Verification items for the finished model (mm, model axes). A direction names the side the tool comes from. Give positions to 0.01 mm unless a question says otherwise; leave off trailing zeros. Loops run counter-clockwise (first coordinate to the right, second up) from the corner with the lowest first, then second, coordinate; pieces in that order, holes last. Notation, with made-up numbers: M 35,77 L 67,77 A22 ccw 67,86 Z; hole C -11,77 d6. An arc over 180 degrees is marked long. Use CSV: the item, a comma, the result in double quotes.
from build123d import *

# Parameters (mm, degrees)
F0_W     = 50.8
F0_H     = 50.8
F0_R     = 9.525
F1_DEPTH = 50.8
F2_DEPTH = 3.175
F3_R     = 2.38125
F4_DEPTH = 25.4
F5_W     = 4.124446
F5_H     = 1.190625
F6_DEPTH = 25.4
F7_R     = 3.175
F8_R     = 0.79375


with BuildPart() as f1:
    # F0 (on Front) → F1 (new body)
    with BuildSketch(Plane.XZ):
        Rectangle(F0_W, F0_H)
        Circle(F0_R, mode=Mode.SUBTRACT)
        Circle(F0_R)
    extrude(amount=-F1_DEPTH)

    # F0 (on Front) → F2 (join)
    with BuildSketch(Plane.XZ):
        Circle(F0_R)
    extrude(amount=F2_DEPTH)

    # F3 (on face) → F4 (join)
    with BuildSketch(Plane.XZ.offset(3.175)):
        Circle(F3_R)
    extrude(amount=F4_DEPTH)

    # F5 (on face) → F6 (cut, through all)
    with BuildSketch(Plane.XZ.offset(28.575)):
        with Locations((0, 1.785938)):
            Rectangle(F5_W, F5_H)
    extrude(amount=-F6_DEPTH, mode=Mode.SUBTRACT)

    # F7
    f7_edges = [f1.edges().sort_by_distance(p)[0] for p in [
        (25.4, 25.4, 25.4),
        (25.4, 25.4, -25.4),
        (-25.4, 25.4, 25.4),
        (-25.4, 25.4, -25.4),
    ]]
    fillet(f7_edges, radius=F7_R)

    # F8
    f8_edges = [f1.edges().sort_by_distance(p)[0] for p in [
        (0, 0, 25.4),
        (0, 50.8, 25.4),
        (-9.525, -3.175, 0),
    ]]
    fillet(f8_edges, radius=F8_R)


solid = f1.part
(1) Scan lines: L1, parallel to Y at x = 12.5, z = 18.5; L2, parallel to Y at x = 3.5, z = -4.5 (3 decimals); L3, parallel to Z at x = 23, y = 17.5. Record each from-to range of solid material in increasing order. Write a range as from..to.
Calculated:
L1,"y = 0..50.8"
L2,"y = -3.175..50.8"
L3,"z = -25.3..25.3"
(2) Section check B-B on z = 0. Record the cut outline in (x, y) (1 decimal).
Calculated:
outline,"M -25.4,0.8 A0.8 ccw -24.6,0 L -9.5,0 L -9.5,-2.4 A0.8 ccw -8.7,-3.2 L -2.4,-3.2 L -2.4,-28.6 L 2.4,-28.6 L 2.4,-3.2 L 8.7,-3.2 A0.8 ccw 9.5,-2.4 L 9.5,0 L 24.6,0 A0.8 ccw 25.4,0.8 L 25.4,50 A0.8 ccw 24.6,50.8 L -24.6,50.8 A0.8 ccw -25.4,50 Z"
(3) Tool access check on faces 1 (the flat face through (0, -16, 1.191)), 2 (the cylindrical face through (-7.559, -1.174, -5.796)), 3 (the flat face through (-25.4, 25, 0)). Record the directions out of +Z, -Z, +X, -X, +Y, -Y that give a thin tool (end or side, any length) a straight path to the whole face; none if there is none.
Calculated:
face 1,"+Z, +X, -X, -Y"
face 2,"-Y"
face 3,"+Z, -Z, -X, +Y, -Y"
(4) Section check C-C on y = -22.5. Record the cut outline in (x, z).
Calculated:
outline,"M -2.06,1.19 A2.38 ccw long 2.06,1.19 Z"
(5) Section check D-D on x = 0. Record the cut outline in (y, z) (1 decimal).
Calculated:
outline,"M -28.6,-2.4 L -3.2,-2.4 L -3.2,-8.7 A0.8 ccw -2.4,-9.5 L 0,-9.5 L 0,-24.6 A0.8 ccw 0.8,-25.4 L 50,-25.4 A0.8 ccw 50.8,-24.6 L 50.8,24.6 A0.8 ccw 50,25.4 L 0.8,25.4 A0.8 ccw 0,24.6 L 0,9.5 L -2.4,9.5 A0.8 ccw -3.2,8.7 L -3.2,1.2 L -28.6,1.2 Z"
(6) Depth check by flat-ended pin: pin 1 Ø1.5 at (y, z) = (-6, 0.5) entering from +X; pin 2 Ø1.2 at (x, y) = (0, -13) entering from +Z; pin 3 Ø12 at (x, z) = (9, -19.5) entering from -Y. Enter the tip coordinate at first touch or a pass-through.
Calculated:
pin 1,"stops at x = 2.38"
pin 2,"stops at z = 1.19"
pin 3,"stops at y = 0"
(7) Section check A-A on x = 20.5. Record the cut outline in (y, z), plus the area to 3 significant figures.
Calculated:
outline,"M 0,-24.61 A0.79 ccw 0.79,-25.4 L 50.01,-25.4 A0.79 ccw 50.8,-24.61 L 50.8,24.61 A0.79 ccw 50.01,25.4 L 0.79,25.4 A0.79 ccw 0,24.61 Z"
area,"2,580 mm²"
